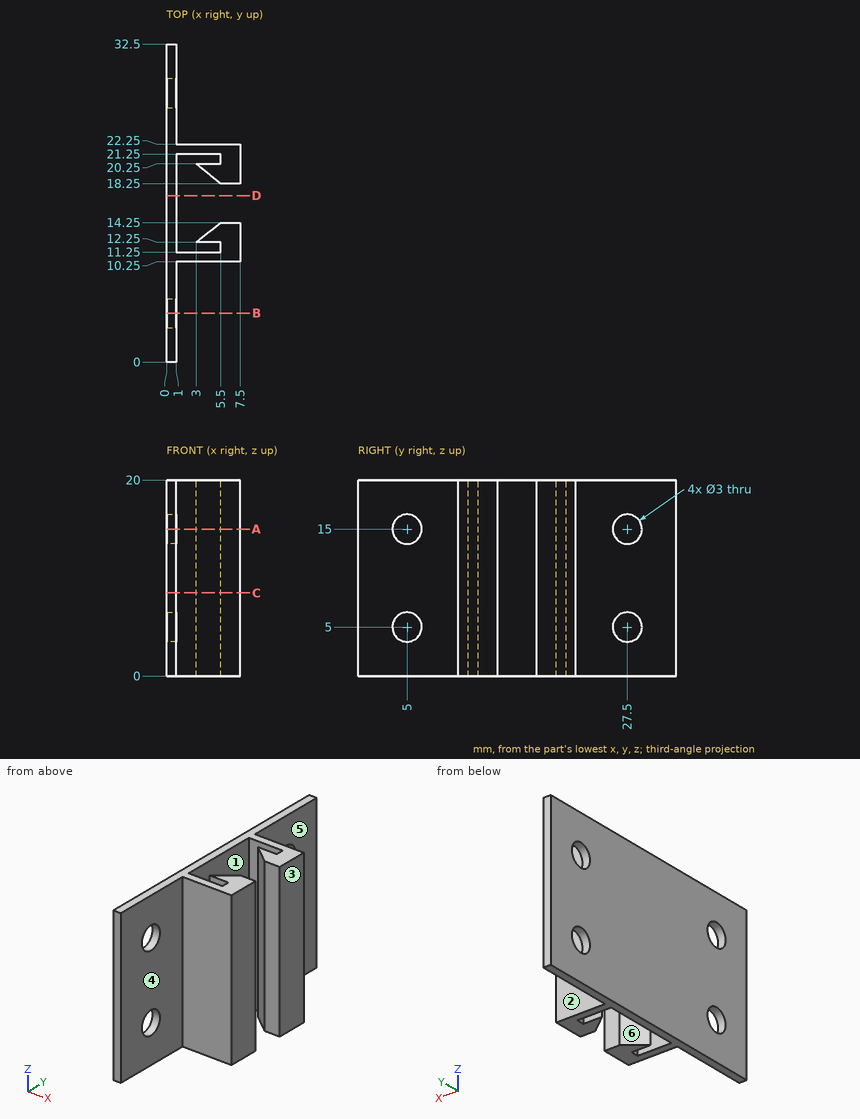
Verification items for this drawing (mm, ordinates from the low corner). A direction names the side the tool comes from. Give positions to 0.01 mm unless a question says otherwise; leave off trailing zeros. Loops run counter-clockwise (first coordinate to the right, second up) from the corner with the lowest first, then second, coordinate; pieces in that order, holes last.
(1) Release check for a two-part mould opening along X. For the marked faces 1, 2 and 3 record: released by +X, released by -X, zero draft, split by the parting line, or undercut.
From the geometry:
face 1: undercut
face 2: zero draft
face 3: released by +X
(2) Set-up check for the marked faces 4, 5 and 6: record each of +Z, -Z, +X, -X, +Y, -Y from which the full face is reachable in a straight line by a thin tool's end or side.
From the geometry:
face 4: +Z, -Z, +X, -Y
face 5: +Z, -Z, +X, +Y
face 6: +Z, -Z
(3) Thickness scan on L1, parallel to Y at x = 0.45, z = 15; L2, parallel to Y at x = 7, z = 18.75; L3, parallel to Y at x = 4.75, z = 17.5. Record the ranges inside material, lowest first.
From the geometry:
L1: y = 0 to 3.5, 6.5 to 26, 29 to 32.5
L2: y = 10.25 to 14.25, 18.25 to 22.25
L3: y = 10.25 to 11.25, 12.25 to 13.65, 18.85 to 20.25, 21.25 to 22.25
(4) Section check B-B on y = 5. Record the cut outline in (x, z), then the cut area to 3 significant figures.
From the geometry:
outline: (0, 0) - (1, 0) - (1, 3.5) - (0, 3.5) - close; (0, 6.5) - (1, 6.5) - (1, 13.5) - (0, 13.5) - close; (0, 16.5) - (1, 16.5) - (1, 20) - (0, 20) - close
area: 14.0 mm2
(5) Section check A-A on z = 15. Record the cut outline in (x, y), then the cut area to 3 significant figures.
From the geometry:
outline: (0, 0) - (1, 0) - (1, 3.5) - (0, 3.5) - close; (0, 6.5) - (1, 6.5) - (1, 10.25) - (7.5, 10.25) - (7.5, 14.25) - (5.5, 14.25) - (3, 12.25) - (5.5, 12.25) - (5.5, 11.25) - (1, 11.25) - (1, 21.25) - (5.5, 21.25) - (5.5, 20.25) - (3, 20.25) - (5.5, 18.25) - (7.5, 18.25) - (7.5, 22.25) - (1, 22.25) - (1, 26) - (0, 26) - close; (0, 29) - (1, 29) - (1, 32.5) - (0, 32.5) - close
area: 56.5 mm2
(6) Section check C-C on z = 8.5. Record the cut outline in (x, y).
From the geometry:
outline: (0, 0) - (1, 0) - (1, 10.25) - (7.5, 10.25) - (7.5, 14.25) - (5.5, 14.25) - (3, 12.25) - (5.5, 12.25) - (5.5, 11.25) - (1, 11.25) - (1, 21.25) - (5.5, 21.25) - (5.5, 20.25) - (3, 20.25) - (5.5, 18.25) - (7.5, 18.25) - (7.5, 22.25) - (1, 22.25) - (1, 32.5) - (0, 32.5) - close
(7) Section check D-D on y = 17. Record the cut outline in (x, z).
From the geometry:
outline: (0, 0) - (1, 0) - (1, 20) - (0, 20) - close
(8) Depth check by flat-ended pin: pin 1 Ø0.5 at (y, z) = (12, 11) entering from -X; pin 2 Ø1.8 at (y, z) = (27.5, 5) entering from -X; pin 3 Ø2 at (x, z) = (4, 14) entering from -Y; pin 4 Ø5 at (y, z) = (5, 15) entering from +X. Enter the tip coordinate at first touch or a pass-through.
From the geometry:
pin 1: stops at x = 0
pin 2: passes through
pin 3: stops at y = 10.25
pin 4: stops at x = 1
